Here's how the part is built. I have some questions about the finished solid (model axes, mm). A direction names the side the tool comes from. Coordinates: 2 decimals unless noted, no trailing zeros. Write each loop counter-clockwise with the first axis right and the second up, starting at its lowest first coordinate (ties: lowest second). Pieces come first, ordered by that corner, then holes.
Item 1: I want a section at C-C (z = 11.75). Please give me the cut outline in (x, y), and give its area (3 significant figures).
Item 2: I want a section at D-D (y = -34). Please give me the cut outline in (x, z).
Item 3: I want a section at B-B (z = 5.5). Count the separate pieces of the cut face and the enclosed holes in it, and give its area (3 significant figures).
Item 4: For faces 1 (the face through (-1.987, -4.734, 4.93)), 2 (the face through (23.797, -5, 5)), 3 (the face through (2, -9.4, 5)), which set-ups out of +Z, -Z, +X, -X, +Y, -Y let a thin tool reach every point of the face, with its end or its side?
Item 5: I'm going to push flat-ended pins straight in: P1, Ø6, axis at x = 19.53, y = -4.72, coming from the +Z side; P2, Ø3.5, axis at x = 3, z = 4.5, coming from the -Y side; P3, Ø7, axis at x = 3.5, z = 4, coming from the -Y side; P4, Ø1.5, axis at x = 16, z = 11.5, coming from the +Y side. Where does each tip first touch, or does it pass through?
Item 6: Please list where these lines run through material, in increasing order: line 1 (X direction, y = -3.5, z = 1); line 2 (X direction, y = -6.5, z = 2); line 3 (Y direction, x = 17.5, z = 9).
Item 7: I want a section at A-A (x = 23). Please give me the cut outline in (y, z).
Item 8: If we mould it in two halves opening along Y, with no side actions, what happens to faces 4 (the face through (-3.54, -0.57, 5.07)), 5 (the face through (18, -9.42, 5)), 6 (the face through (-4.142, -5, 5))? For each: pulls with the +Y half, pulls with the -Y half, needs draft (parallel to the pull), parting line crosses it, or undercut.
Autodesk Inventor part; units mm, degrees
ref_plane "YZ Plane" through (0, 0, 0) normal (1, 0, 0) x (0, 1, 0)
ref_plane "XZ Plane" through (0, 0, 0) normal (0, 1, 0) x (-1, 0, 0)
ref_plane "XY Plane" through (0, 0, 0) normal (0, 0, 1) x (1, 0, 0)
sketch "スケッチ1" plane through (0, 0, 0) normal (0, 0, 1) x (1, 0, 0)
  line L0 (18.408, 0) -> (-1.0303, 0)
  arc A0 (36.165, -44.7764) -> (37.2594, -44.8743) centre (37.0041, -41.5628) ccw
  line L1 (38.972, -43.427) -> (37.2594, -44.8743)
  line L2 (31.483, -28.9072) -> (15.1835, -9.4196)
  circle A1 centre (19.5337, -4.7196) radius 2.5
  line L3 (8.0337, -1.575) -> (1.1379, -1.575)
  arc A2 (7.8277, -7.8182) -> (8.0337, -1.575) centre (8.0337, -4.7) ccw
  line L4 (7.8277, -7.8182) -> (1.0695, -7.8243)
  arc A3 (1.1379, -1.575) -> (1.0695, -7.8243) centre (1.1379, -4.7) ccw
  line L5 (36.165, -44.7764) -> (6.576, -9.4)
  line L6 (18.408, 0) -> (23.7968, 0)
  line L7 (23.7968, 0) -> (23.7968, -8.35)
  line L8 (-1.0303, 0) -> (-4.1421, 0)
  line L9 (-4.1421, 0) -> (-4.1421, -7.7348)
  line L10 (-4.1421, -7.7348) -> (-4.1421, -9.4)
  line L11 (-4.1421, -9.4) -> (6.576, -9.4)
  line L12 (15.1835, -9.4196) -> (23.7968, -9.4196)
  line L13 (23.7968, -9.4196) -> (23.7968, -7.7545)
  line L14 (41.7112, -41.1359) -> (41.7109, -41.1356)
  line L15 (41.7109, -41.1356) -> (43.7109, -39.4628)
  line L16 (43.7109, -39.4628) -> (30.8794, -24.1216)
  line L17 (30.8794, -24.1216) -> (28.8794, -25.7944)
  line L18 (38.972, -43.427) -> (41.7112, -41.1359)
  line L19 (31.483, -28.9072) -> (41.7112, -41.1359)
  point P0 (0, 0)
  point P1 (0, 0)
  dimension "d0" = 5
  dimension "d1" = 3.125
  dimension "d3" = 11.5
  dimension "d5" = 4.7
  dimension "d9" = 3.125
  dimension "d11" = 4.7
  dimension "d12" = 4.7
  dimension "d13" = 6.8958
  dimension "d14" = 20
  dimension "d19" = 2
  dimension "d24" = 46.1194
  dimension "d25" = 41.3474
extrude "押し出し1" add sketch "スケッチ1" along normal blind 10
fillet "フィレット1" radius 2 4 edges at (23.7968, 0, 5) (23.7968, -9.4196, 5) (-4.1421, 0, 5) (-4.1421, -9.4, 5)
fillet "フィレット2" radius 2 2 edges at (37.2594, -44.8743, 5) (36.165, -44.7764, 5)
sketch "スケッチ4" plane through (0, 0, 10) normal (0, 0, 1) x (1, 0, 0)
  line L0 (30.8794, -24.1216) -> (28.8794, -25.7944)
  line L1 (43.7109, -39.4628) -> (30.8794, -24.1216)
  line L2 (41.7109, -41.1356) -> (43.7109, -39.4628)
  line L3 (28.8794, -25.7944) -> (41.7109, -41.1356)
  line L4 (43.7109, -39.4628) -> (41.7109, -41.1356)
  line L5 (28.8794, -25.7944) -> (30.8794, -24.1216)
  line L6 (30.8794, -24.1216) -> (43.7109, -39.4628)
  point P0 (0, 0)
extrude "押し出し4" add sketch "スケッチ4" along normal blind 5
equation "\"d5\" = d11"
equation "\"d9\" = d1"
properties part number "finger_3"
Answer:
1. outline: (28.88, -25.79) - (41.71, -41.14) - (43.71, -39.46) - (30.88, -24.12) - close
1. area: 52.1 mm2
2. outline: (27.15, 0) - (39.14, 0) - (39.14, 15) - (35.74, 15) - (35.74, 10) - (27.15, 10) - close
3. separate pieces: 1
3. enclosed holes: 2
3. area: 508 mm2
4. face 1: +Z, -Z
4. face 2: +Z, -Z, +X, +Y
4. face 3: +Z, -Z, -X, -Y
5. P1: stops at z = 10
5. P2: stops at y = -9.4
5. P3: stops at y = -9.91
5. P4: passes through
6. line 1: x = -4.14 to -1.75, 10.92 to 17.35, 21.72 to 23.8
6. line 2: x = -4.14 to -1.42, 10.59 to 17.78, 21.29 to 23.8
6. line 3: y = -22.46 to -12.19, -9.42 to -6.17, -3.27 to 0
7. outline: (-29.04, 0) - (-18.76, 0) - (-18.76, 10) - (-29.04, 10) - close; (-9.02, 0) - (-0.4, 0) - (-0.4, 10) - (-9.02, 10) - close
8. face 4: pulls with the +Y half
8. face 5: undercut
8. face 6: needs draft
